Read the model definition and answer for the solid it produces. Units are mm, in the model's axes. Face numbers are marked on the shaded views. A direction names the side the tool comes from. Give positions to 0.01 mm unless a question says otherwise; leave off trailing zeros. Write each loop counter-clockwise with the first axis right and the second up, starting at its lowest first coordinate (ties: lowest second). Pieces come first, ordered by that corner, then holes. Notation, with made-up numbers: M -13.5,-7 L 30.5,-7 A13 cw 30.5,2 Z; hole C -4,52 d11. An arc over 180 degrees is marked long. Put each result on its own line as item: value.
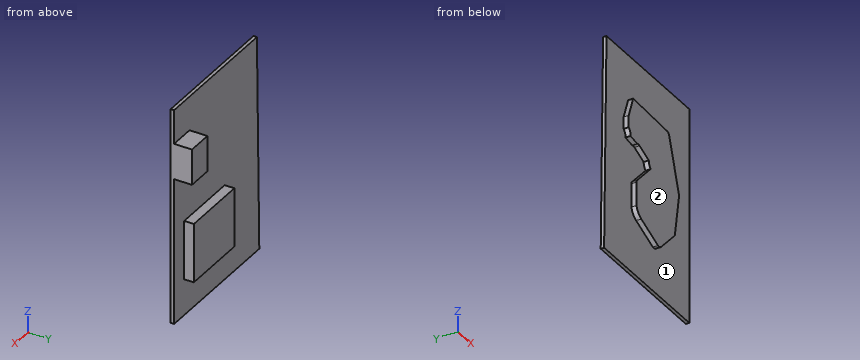
Autodesk Inventor part; units mm, degrees
ref_plane "YZ Plane" through (0, 0, 0) normal (1, 0, 0) x (0, 1, 0)
ref_plane "XZ Plane" through (0, 0, 0) normal (0, 1, 0) x (-1, 0, 0)
ref_plane "XY Plane" through (0, 0, 0) normal (0, 0, 1) x (1, 0, 0)
sketch "Sketch1" plane through (0, 0, 0) normal (0, 1, 0) x (-1, 0, 0)
  line L0 (0, 0) -> (24.2, 0)
  line L1 (24.2, 0) -> (24.9, -38.1436)
  line L2 (24.9, -38.1436) -> (0, -38.1436)
  line L3 (0, -38.1436) -> (0, 0)
  dimension "d0" = 38.15
  dimension "d1" = 24.9
  dimension "d2" = 24.2
extrude "Extrusion1" add sketch "Sketch1" along normal blind 0.6
sketch "Sketch2" plane through (0, 0.6, 0) normal (0, 1, 0) x (1, 0, 0)
  line L0 (0, 38.1436) -> (-24.9, 38.1436)
  line L1 (-24.9, 38.1436) -> (-24.2, 0)
  line L2 (-24.2, 0) -> (0, 0)
  line L3 (0, 0) -> (0, 38.1436)
  line L4 (0, 6) -> (-4.5, 6)
  line L5 (-4.5, 6) -> (-4.5, 12.3)
  line L6 (-4.5, 12.3) -> (0, 12.3)
  line L7 (0, 12.3) -> (0, 6)
  point P0 (0, 12.3)
  dimension "d5" = 4.5
  dimension "d6" = 6.3
  dimension "d7" = 6
  dimension "d8" = 25.8436
extrude "Extrusion2" add sketch "Sketch2" along normal blind 3.15 contours L3 L4 L5 L6
sketch "Sketch3" plane through (0, 0.6, 0) normal (0, 1, 0) x (1, 0, 0)
  line L0 (-14.7887, 21.3392) -> (-2.9463, 21.3392)
  line L1 (-2.9463, 21.3392) -> (-2.9463, 31.7514)
  line L2 (-2.9463, 31.7514) -> (-14.7887, 31.7514)
  line L3 (-14.7887, 31.7514) -> (-14.7887, 21.3392)
  point P0 (0, 0)
extrude "Extrusion3" add sketch "Sketch3" along normal blind 1.7
sketch "Sketch4" plane through (0, 0, 0) normal (0, -1, 0) x (1, 0, 0)
  line L0 (-17.8896, -8.0503) -> (-7.9992, -8.5103)
  arc A0 (-7.4114, -8.8426) -> (-7.9992, -8.5103) centre (-8.034, -9.258) ccw
  line L1 (-7.4114, -8.8426) -> (-4.5491, -17.8896)
  arc A1 (-4.5491, -18.6308) -> (-4.5491, -17.8896) centre (-5.7203, -18.2602) ccw
  line L2 (-4.5491, -18.6308) -> (-5.7203, -25.9399)
  arc A2 (-5.7203, -25.9399) -> (-5.7203, -25.9399) centre (-3.4138, -26.3096) ccw
  line L3 (-5.7203, -25.9399) -> (-9.7115, -30.1057)
  arc A3 (-10.6571, -30.3612) -> (-9.7115, -30.1057) centre (-10.3961, -29.4497) ccw
  line L4 (-10.6571, -30.3612) -> (-15.5384, -28.2656)
  arc A4 (-16.9185, -26.6044) -> (-15.5384, -28.2656) centre (-14.6016, -26.0835) ccw
  line L5 (-16.9185, -26.6044) -> (-16.9185, -22.4387)
  arc A5 (-16.6885, -21.9531) -> (-16.9185, -22.4387) centre (-16.2909, -22.4387) ccw
  line L6 (-16.6885, -21.9531) -> (-12.7952, -17.8896)
  arc A6 (-13.3329, -16.6318) -> (-12.7952, -17.8896) centre (-11.5884, -16.63) ccw
  line L7 (-13.3329, -16.6318) -> (-16.0354, -15.4715)
  arc A7 (-16.0354, -15.4715) -> (-16.6885, -15.4715) centre (-16.3619, -16.2321) ccw
  line L8 (-16.6885, -15.4715) -> (-18.6774, -15.1528)
  arc A8 (-18.6774, -15.1528) -> (-19.193, -13.8772) centre (-19.9919, -14.9421) ccw
  line L9 (-19.193, -13.8772) -> (-19.193, -11.7599)
  line L10 (-19.193, -11.7599) -> (-17.8896, -8.0503)
  point P0 (0, 0)
extrude "Extrusion4" add sketch "Sketch4" along normal blind 0.9 contours L0 A0 L1 A1 L2 L3 A3 L4 A4 L5 A5 L6 A6 L7 A7 L8 A8 L9 L10
properties part number "adc"
(1) Section D-D on x = -20.5 is taken. Determine the outline of the cut face in (y, z), and give its area (3 significant figures).
Result:
outline: M 0,-38.14 L 0.6,-38.14 L 0.6,0 L 0,0 Z
area: 22.9 mm²
(2) Section A-A on y = 1.05 is taken. Determine the outline of the cut face in (x, z).
Result:
outline: M -14.79,-31.75 L -2.95,-31.75 L -2.95,-21.34 L -14.79,-21.34 Z; M -4.5,-12.3 L 0,-12.3 L 0,-6 L -4.5,-6 Z
(3) Section B-B on x = -2.25 is taken. Determine the outline of the cut face in (y, z), and give its area (3 significant figures).
Result:
outline: M 0,-38.14 L 0.6,-38.14 L 0.6,-12.3 L 3.75,-12.3 L 3.75,-6 L 0.6,-6 L 0.6,0 L 0,0 Z
area: 42.7 mm²
(4) Section C-C on y = 2.85 is taken. Determine the outline of the cut face in (x, z).
Result:
outline: M -4.5,-12.3 L 0,-12.3 L 0,-6 L -4.5,-6 Z
(5) Straight lines are drawn through the part: line 1 along X through (y, z) = (2, -23); line 2 along Y through (x, z) = (-12.25, -30.5); line 3 along Z through (x, y) = (-9, 1.65). For each, find the intervals that lie inside material, in ascending order. Write a range as from..to.
Result:
line 1: x = -14.79..-2.95
line 2: y = 0..2.3
line 3: z = -31.75..-21.34
(6) Which of the six approach directions +Z, -Z, +X, -X, +Y, -Y give full straight-line access (tool end or side, diameter ignored) to the marked faces 1 and 2?
Result:
face 1: -Y
face 2: +Z, -Z, +X, -X, -Y
(7) Given pin 1 Ø0.9 at (x, y) = (-2.5, 1.5) entering from +Z; pin 2 Ø2 at (y, z) = (2.5, -28) entering from +X; pin 3 Ø0.5 at (x, y) = (-9.5, 2) entering from -Z, each flat-ended and moving along its own axis, determine where each tip first touches the part or whether it passes through.
Result:
pin 1: stops at z = -6
pin 2: stops at x = -2.95
pin 3: stops at z = -31.75
